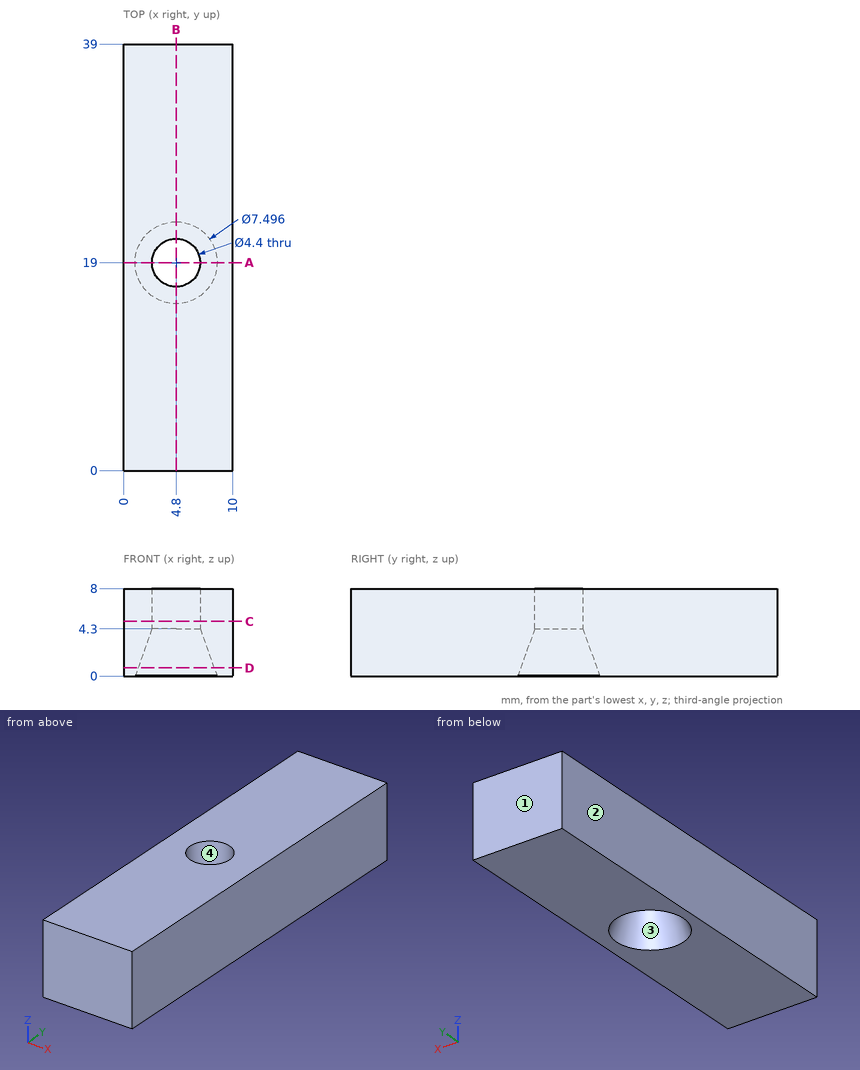
Verification items for this drawing (mm, ordinates from the low corner). Coordinates: 2 decimals unless noted, no trailing zeros. Write each loop counter-clockwise with the first axis right and the second up, starting at its lowest first coordinate (ties: lowest second). Pieces come first, ordered by that corner, then holes. Notation, with made-up numbers: (57.5, 11.5) -> (91.5, 11.5) arc R30 cw to (91.5, 43.5) -> close; hole circle Ø1 at (82.5, 11). An arc over 180 degrees is marked (long way). One line per item, written item: value. Start each with the question number.
Q1. Cross-section at A-A on y = 19. Enter the section's corners in (x, z).
Q2. Mould release check, pull along X, two halves, no side actions. Record for the marked faces 1, 2, 3 and 4: pulls with the +X half, pulls with the -X half, needs draft (parallel to the pull), parting line crosses it, or undercut.
Q3. Cross-section at B-B on x = 4.8. Enter the section's corners in (y, z).
Q4. Thickness scan on L1, parallel to X at y = 19, z = 5.3; L2, parallel to Y at x = 5, z = 4.5; L3, parallel to Y at x = 4.5, z = 4. Record the ranges inside material, lowest first. Write a range as from..to.
Q5. Cross-section at C-C on z = 5. Enter the section's corners in (x, y), and give its area (3 significant figures).
Q6. Cross-section at D-D on z = 0.75. Enter the section's corners in (x, y).
Checked values:
1. outline: (0, 0) -> (1.05, 0) -> (2.6, 4.3) -> (2.6, 8) -> (0, 8) -> close; (7, 4.3) -> (8.55, 0) -> (10, 0) -> (10, 8) -> (7, 8) -> close
2. face 1: needs draft
2. face 2: pulls with the -X half
2. face 3: undercut
2. face 4: undercut
3. outline: (0, 0) -> (15.25, 0) -> (16.8, 4.3) -> (16.8, 8) -> (0, 8) -> close; (21.2, 4.3) -> (22.75, 0) -> (39, 0) -> (39, 8) -> (21.2, 8) -> close
4. L1: x = 0..2.6, 7..10
4. L2: y = 0..16.81, 21.19..39
4. L3: y = 0..16.71, 21.29..39
5. outline: (0, 0) -> (10, 0) -> (10, 39) -> (0, 39) -> close; hole circle Ø4.4 at (4.8, 19)
5. area: 375 mm²
6. outline: (0, 0) -> (10, 0) -> (10, 39) -> (0, 39) -> close; hole circle Ø6.96 at (4.8, 19)
